Check sheet for the modelled part. Datum: model origin and axes. Units: mm. A direction names the side the tool comes from. Give positions to 0.01 mm unless a question says otherwise; leave off trailing zeros. Write each loop counter-clockwise with the first axis right and the second up, starting at its lowest first coordinate (ties: lowest second). Pieces come first, ordered by that corner, then holes. Notation, with made-up numbers: (-6, 63) -> (32, 63) arc R14 cw to (32, 86) -> close; hole circle Ø9 at (40.5, 20). An arc over 180 degrees is marked (long way). Use a Markdown table: item, result. Add a question column.
1. Set-up check for faces 1 (the flat face through (10, -4, -15)), 2 (the flat face through (15, -250, 0)), 3 (the flat face through (20, -4, 15)), 4 (the flat face through (20, -4, -15)): record each of +Z, -Z, +X, -X, +Y, -Y from which the full face is reachable in a straight line by a thin tool's end or side.
2. Cross-section at B-B (y = 192). Enter the section's corners in (x, z), then the cut area to 3 significant figures.
3. Gauge pin test, flat ends, axial feed: P1, Ø5, axis at y = 13, z = -16, coming from the +X side; P2, Ø5, axis at x = 16.5, y = -39, coming from the +Z side; P3, Ø3, axis at x = 25.5, y = 12.5, coming from the -Z side. Record the tip position at first contact, or that the pin passes through.
4. Cross-section at A-A (x = 5.25). Enter the section's corners in (y, z), then the cut area to 3 significant figures.
5. Scan lines: probe 1 along X at (y, z) = (-157, 17.5); probe 2 along Z at (x, y) = (9.25, -235); probe 3 along Z at (x, y) = (8.75, -30). Record each from-to range of solid material in increasing order. Write a range as [from, to].
from build123d import *

# Parameters (mm, degrees)
F0_W     = 500
F0_H     = 20
F1_DEPTH = 30
F2_W     = 10
F2_H     = 10
F3_DEPTH = 500
F4_W     = 10
F4_H     = 10
F5_DEPTH = 500
F6_W     = 10
F6_H     = 10
F7_DEPTH = 500
F8_R     = 3
F9_DEPTH = 30


with BuildPart() as f1:
    # F0 (on Right) → F1 (new body)
    with BuildSketch(Plane.YZ):
        Rectangle(F0_W, F0_H)
    extrude(amount=F1_DEPTH)

    # F2 (on face) → F3 (join)
    with BuildSketch(Plane.XZ.offset(250)):
        with Locations((5, 15)):
            Rectangle(F2_W, F2_H)
    extrude(amount=-F3_DEPTH)

    # F4 (on face) → F5 (join)
    with BuildSketch(Plane.XZ.offset(250)):
        with Locations((25, 15)):
            Rectangle(F4_W, F4_H)
    extrude(amount=-F5_DEPTH)

    # F6 (on face) → F7 (join)
    with BuildSketch(Plane.XZ.offset(250)):
        with Locations((15, -15)):
            Rectangle(F6_W, F6_H)
    extrude(amount=-F7_DEPTH)

    # F8 (on face) → F9 (cut)
    with BuildSketch(Plane.YZ.offset(30)):
        with Locations((-235, 0)):
            Circle(F8_R)
        with Locations((235, 0)):
            Circle(F8_R)
    extrude(amount=-F9_DEPTH, mode=Mode.SUBTRACT)


solid = f1.part
Worked answers:
| question | item | result |
|---|---|---|
| 1 | face 1 | -Z, -X, +Y, -Y |
| 1 | face 2 | +Z, -Z, +X, -X, -Y |
| 1 | face 3 | +Z, +Y, -Y |
| 1 | face 4 | -Z, +X, +Y, -Y |
| 2 | outline | (0, -10) -> (10, -10) -> (10, -20) -> (20, -20) -> (20, -10) -> (30, -10) -> (30, 20) -> (20, 20) -> (20, 10) -> (10, 10) -> (10, 20) -> (0, 20) -> close |
| 2 | area | 900 mm² |
| 3 | P1 | stops at x = 20 |
| 3 | P2 | stops at z = 10 |
| 3 | P3 | stops at z = -10 |
| 4 | outline | (-250, -10) -> (250, -10) -> (250, 20) -> (-250, 20) -> close; hole circle Ø6 at (-235, 0); hole circle Ø6 at (235, 0) |
| 4 | area | 14,900 mm² |
| 5 | probe 1 | x = [0, 10], [20, 30] |
| 5 | probe 2 | z = [-10, -3], [3, 20] |
| 5 | probe 3 | z = [-10, 20] |
